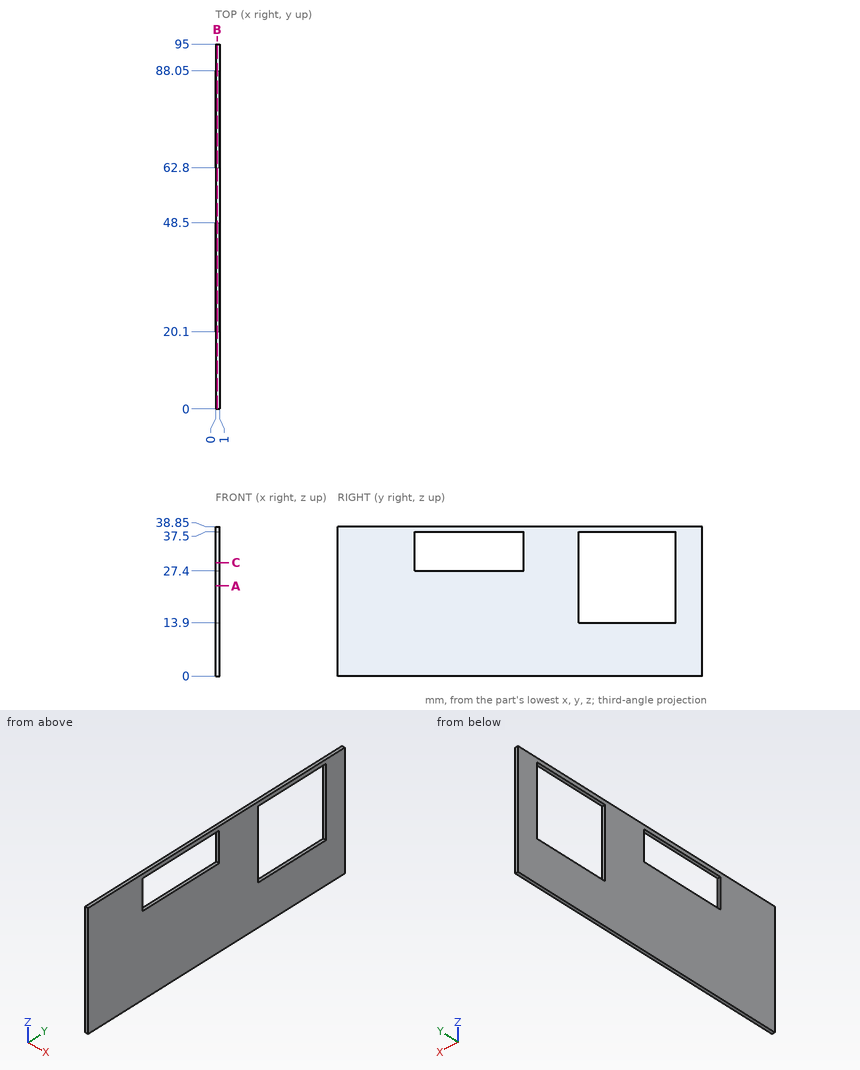
Answer from the drawing. Dimensions are ordinates in mm from the lowest x, y and z of the part. Give positions to 0.01 mm unless a question says otherwise; leave off trailing zeros. Order: outer loops, then holes, each group sorted by start corner. A loop starts at its lowest first (then second) coordinate and runs counter-clockwise, first axis right, second up. Notation, with made-up numbers: (61, 72.5) -> (86, 72.5) arc R22 cw to (86, 92.5) -> close; hole circle Ø1 at (84.5, 70). An arc over 180 degrees is marked (long way). One line per item, written item: value. Start each with the question number.
(1) The part is cut by section B-B (x = 0.4). Determine the outline of the cut face in (y, z), and give its area (3 significant figures).
(2) The part is cut by section C-C (z = 29.5). Determine the outline of the cut face in (x, y), and give its area (4 significant figures).
(3) Straight lines are drawn through the part: L1, parallel to Y at x = 0.2, z = 34; L2, parallel to Y at x = 0.9, z = 27; L3, parallel to Z at x = 0.05, y = 40.5. For each, find the intervals that lie inside material, in ascending order.
(4) The part is cut by section A-A (z = 23.5). Determine the outline of the cut face in (x, y), and give its area (4 significant figures).
Taken from the geometry:
1. outline: (0, 0) -> (95, 0) -> (95, 38.85) -> (0, 38.85) -> close; hole (20.1, 27.4) -> (48.5, 27.4) -> (48.5, 37.5) -> (20.1, 37.5) -> close; hole (62.8, 13.9) -> (88.05, 13.9) -> (88.05, 37.5) -> (62.8, 37.5) -> close
1. area: 2,810 mm^2
2. outline: (0, 0) -> (1, 0) -> (1, 20.1) -> (0, 20.1) -> close; (0, 48.5) -> (1, 48.5) -> (1, 62.8) -> (0, 62.8) -> close; (0, 88.05) -> (1, 88.05) -> (1, 95) -> (0, 95) -> close
2. area: 41.35 mm^2
3. L1: 0 to 20.1, 48.5 to 62.8, 88.05 to 95
3. L2: 0 to 62.8, 88.05 to 95
3. L3: 0 to 27.4, 37.5 to 38.85
4. outline: (0, 0) -> (1, 0) -> (1, 62.8) -> (0, 62.8) -> close; (0, 88.05) -> (1, 88.05) -> (1, 95) -> (0, 95) -> close
4. area: 69.75 mm^2
